Could you check a few things on this model? Use its own coordinates, in mm. Face numbers are marked on the shaded views. A direction names the side the tool comes from. Round coordinates to 2 decimals unless told otherwise and drop trailing zeros. Order: outer loops, then holes, each group sorted by start corner. A loop starts at its lowest first (then second) coordinate and runs counter-clockwise, first axis right, second up. Notation, with made-up numbers: (19, 89) - (71, 89) arc R27 ccw to (71, 123) - close; hole circle Ø6 at (56.5, 28). An arc over 180 degrees is marked (long way). Use one line per item in the form item = value.
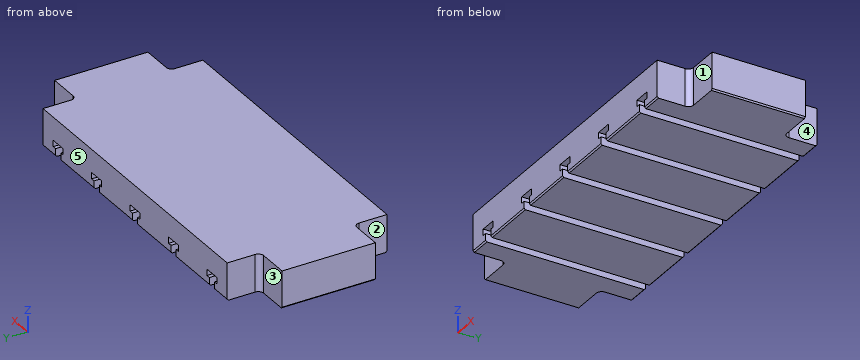
from build123d import *

# Parameters (mm, degrees)
F0_W     = 901.7
F0_H     = 381
F1_DEPTH = 88.9
F2_SIZE  = 3.175
F4_DEPTH = 381.001
F6_DEPTH = 88.901
F8_ANGLE = 180


with BuildPart() as f1:
    # F0 (on Top) → F1 (new body)
    with BuildSketch(Plane.XY):
        Rectangle(F0_W, F0_H)
    extrude(amount=F1_DEPTH)

    # F2
    f2_edges = [f1.edges().sort_by_distance(p)[0] for p in [
        (0, -190.5, 88.9),
        (450.85, 0, 88.9),
        (0, 190.5, 88.9),
        (-450.85, 0, 88.9),
    ]]
    chamfer(f2_edges, length=F2_SIZE)

    # F3 (on face) → F4 (cut, through all)
    with BuildSketch(Plane.XZ.offset(190.5)):
        Polygon((315.11875, 88.9), (294.48125, 88.9), (294.48125, 69.85), (284.95625, 69.85), (284.95625, 54.76875), (324.64375, 54.76875), (324.64375, 69.85), (315.11875, 69.85), align=None)
        Polygon((162.71875, 88.9), (142.08125, 88.9), (142.08125, 69.85), (132.55625, 69.85), (132.55625, 54.76875), (172.24375, 54.76875), (172.24375, 69.85), (162.71875, 69.85), align=None)
        Polygon((10.31875, 88.9), (-10.31875, 88.9), (-10.31875, 69.85), (-19.84375, 69.85), (-19.84375, 54.76875), (19.84375, 54.76875), (19.84375, 69.85), (10.31875, 69.85), align=None)
        Polygon((-142.08125, 88.9), (-162.71875, 88.9), (-162.71875, 69.85), (-172.24375, 69.85), (-172.24375, 54.76875), (-132.55625, 54.76875), (-132.55625, 69.85), (-142.08125, 69.85), align=None)
        Polygon((-294.48125, 88.9), (-315.11875, 88.9), (-315.11875, 69.85), (-324.64375, 69.85), (-324.64375, 54.76875), (-284.95625, 54.76875), (-284.95625, 69.85), (-294.48125, 69.85), align=None)
    extrude(amount=-F4_DEPTH, mode=Mode.SUBTRACT)

    # F5 (on face) → F6 (cut, through all)
    with BuildSketch(Plane(origin=(0, 0, 0), x_dir=(1, 0, 0), z_dir=(0, 0, -1))):
        with BuildLine():
            Line((-450.85, -190.5), (-365.125, -190.5))
            Line((-365.125, -190.5), (-365.125, -123.825))
            ThreePointArc((-365.125, -123.825), (-368.844744, -114.844744), (-377.825, -111.125))
            Line((-377.825, -111.125), (-450.85, -111.125))
            Line((-450.85, -111.125), (-450.85, -190.5))
        make_face()
        with BuildLine():
            ThreePointArc((377.825, -111.125), (368.844744, -114.844744), (365.125, -123.825))
            Line((365.125, -123.825), (365.125, -190.5))
            Line((365.125, -190.5), (450.85, -190.5))
            Line((450.85, -190.5), (450.85, -111.125))
            Line((450.85, -111.125), (377.825, -111.125))
        make_face()
        with BuildLine():
            Line((365.125, 190.5), (365.125, 123.825))
            ThreePointArc((365.125, 123.825), (368.844744, 114.844744), (377.825, 111.125))
            Line((377.825, 111.125), (450.85, 111.125))
            Line((450.85, 111.125), (450.85, 190.5))
            Line((450.85, 190.5), (365.125, 190.5))
        make_face()
        with BuildLine():
            ThreePointArc((-377.825, 111.125), (-368.844744, 114.844744), (-365.125, 123.825))
            Line((-365.125, 123.825), (-365.125, 190.5))
            Line((-365.125, 190.5), (-450.85, 190.5))
            Line((-450.85, 190.5), (-450.85, 111.125))
            Line((-450.85, 111.125), (-377.825, 111.125))
        make_face()
    extrude(amount=-F6_DEPTH, mode=Mode.SUBTRACT)


with BuildPart() as f1_1:
    # F8: moved
    add(f1.part.rotate(Axis((1.057014, 0, 0), (1, 0, 0)), F8_ANGLE))


solid = f1_1.part
Item 1: For the marked faces 1, 2, 3, 4 and 5, which set-ups out of +Z, -Z, +X, -X, +Y, -Y let a thin tool reach every point of the face, with its end or its side?
Found:
face_1 = +Z, -Z, +X, -Y
face_2 = +Z, -Z, -X, -Y
face_3 = +Z, -Z, -X, +Y
face_4 = +Z, -Z, +X, +Y
face_5 = +Z, -Z, +X, -X, +Y
Item 2: Imagine slicing it at A-A on z = -34. Please give me the cut outline in (x, y) (3 decimals), plus the area to 3 significant figures.
Found:
outline = (-450.85, -111.125) - (-377.825, -111.125) arc R12.7 cw to (-365.125, -123.825) - (-365.125, -190.5) - (365.125, -190.5) - (365.125, -123.825) arc R12.7 cw to (377.825, -111.125) - (450.85, -111.125) - (450.85, 111.125) - (377.825, 111.125) arc R12.7 cw to (365.125, 123.825) - (365.125, 190.5) - (-365.125, 190.5) - (-365.125, 123.825) arc R12.7 cw to (-377.825, 111.125) - (-450.85, 111.125) - close
area = 316,000 mm2
Item 3: I need wall thicknesses on L1, parallel to X at y = 139.5, z = -68.5 (3 decimals); L2, parallel to X at y = 42.5, z = -62.5; L3, parallel to Z at x = -286, y = 17.5. Which ranges of each line are inside material? Lowest first, please.
Found:
L1 = -365.125 to -324.644, -284.956 to -172.244, -132.556 to -19.844, 19.844 to 132.556, 172.244 to 284.956, 324.644 to 365.125
L2 = -450.85 to -324.64, -284.96 to -172.24, -132.56 to -19.84, 19.84 to 132.56, 172.24 to 284.96, 324.64 to 450.85
L3 = -88.9 to -69.85, -54.77 to 0
Item 4: Will this pin go through, and if not, where does the flat tip stop? P1, Ø10, axis at y = -122.5, z = -70.5, coming from the +X side.
Found:
P1 = 366.81
